```python
from build123d import *

# Parameters (mm, degrees)
BOSS_EXTRUDE1_DEPTH = 1.1
SKETCH3_W           = 2.15
SKETCH3_H           = 30
SKETCH4_W           = 2.15
SKETCH4_H           = 30
SKETCH5_R           = 1.5
CUT_EXTRUDE1_DEPTH  = 28


with BuildPart() as part:
    # Sketch2 → Boss-Extrude1 (new body)
    with BuildSketch(Plane.XY):
        with BuildLine():
            Line((-20.5, -0.55), (-13.5, -0.55))
            ThreePointArc((-13.5, -0.55), (-12.403984489, -0.096015511), (-11.95, 1))
            Line((-11.95, 1), (-11.95, 7))
            ThreePointArc((-11.95, 7), (-11, 7.95), (-10.05, 7))
            Line((-10.05, 7), (-10.05, 0))
            Line((-10.05, 0), (-10.05, -7))
            ThreePointArc((-10.05, -7), (-8, -9.05), (-5.95, -7))
            Line((-5.95, -7), (-5.95, 0))
            Line((-5.95, 0), (-5.95, 7))
            ThreePointArc((-5.95, 7), (-5, 7.95), (-4.05, 7))
            Line((-4.05, 7), (-4.05, 0))
            Line((-4.05, 0), (-4.05, -7))
            ThreePointArc((-4.05, -7), (-2, -9.05), (0.05, -7))
            Line((0.05, -7), (0.05, 0))
            Line((0.05, 0), (0.05, 7))
            ThreePointArc((0.05, 7), (1, 7.95), (1.95, 7))
            Line((1.95, 7), (1.95, 0))
            Line((1.95, 0), (1.95, -7))
            ThreePointArc((1.95, -7), (4, -9.05), (6.05, -7))
            Line((6.05, -7), (6.05, -1))
            ThreePointArc((6.05, -1), (6.181801948, -0.681801948), (6.5, -0.55))
            Line((6.5, -0.55), (13.5, -0.55))
            ThreePointArc((13.5, -0.55), (14.05, 0), (13.5, 0.55))
            Line((13.5, 0.55), (6.5, 0.55))
            ThreePointArc((6.5, 0.55), (5.403984489, 0.096015511), (4.95, -1))
            Line((4.95, -1), (4.95, -7))
            ThreePointArc((4.95, -7), (4, -7.95), (3.05, -7))
            Line((3.05, -7), (3.05, 0))
            Line((3.05, 0), (3.05, 7))
            ThreePointArc((3.05, 7), (1, 9.05), (-1.05, 7))
            Line((-1.05, 7), (-1.05, 0))
            Line((-1.05, 0), (-1.05, -7))
            ThreePointArc((-1.05, -7), (-2, -7.95), (-2.95, -7))
            Line((-2.95, -7), (-2.95, 0))
            Line((-2.95, 0), (-2.95, 7))
            ThreePointArc((-2.95, 7), (-5, 9.05), (-7.05, 7))
            Line((-7.05, 7), (-7.05, 0))
            Line((-7.05, 0), (-7.05, -7))
            ThreePointArc((-7.05, -7), (-8, -7.95), (-8.95, -7))
            Line((-8.95, -7), (-8.95, 0))
            Line((-8.95, 0), (-8.95, 7))
            ThreePointArc((-8.95, 7), (-11, 9.05), (-13.05, 7))
            Line((-13.05, 7), (-13.05, 1))
            ThreePointArc((-13.05, 1), (-13.181801948, 0.681801948), (-13.5, 0.55))
            Line((-13.5, 0.55), (-20.5, 0.55))
            ThreePointArc((-20.5, 0.55), (-21.05, 0), (-20.5, -0.55))
        make_face()
    extrude(amount=BOSS_EXTRUDE1_DEPTH)

    # Sketch3 → Revolve1 (revolve)
    with BuildSketch(Plane(origin=(0, 0, 0), x_dir=(-1, 0, 0), z_dir=(0, -1, 0)), mode=Mode.PRIVATE) as revolve1_sk:
        with Locations((21.575, 13.9)):
            Rectangle(SKETCH3_W, SKETCH3_H)
    revolve(revolve1_sk.sketch.rotate(Axis((-20.5, 0, 1.1), (0, 0, -1)), 180), axis=Axis((-20.5, 0, 1.1), (0, 0, -1)))

    # Sketch4 → Revolve2 (revolve)
    with BuildSketch(Plane(origin=(0, 0, 0), x_dir=(-1, 0, 0), z_dir=(0, -1, 0)), mode=Mode.PRIVATE) as revolve2_sk:
        with Locations((-14.575, 13.9)):
            Rectangle(SKETCH4_W, SKETCH4_H)
    revolve(revolve2_sk.sketch.rotate(Axis((13.5, 0, -28.9), (0, 0, 1)), 180), axis=Axis((13.5, 0, -28.9), (0, 0, 1)))

    # Sketch5 → Cut-Extrude1 (cut)
    with BuildSketch(Plane(origin=(0, 0, -28.9), x_dir=(-1, 0, 0), z_dir=(0, 0, -1))):
        with Locations((20.5, 0)):
            Circle(SKETCH5_R)
        with Locations((-13.5, 0)):
            Circle(SKETCH5_R)
    extrude(amount=-CUT_EXTRUDE1_DEPTH, mode=Mode.SUBTRACT)


solid = part.part
```
Can you work these out from the model? Positions are in its coordinate system, mm. A direction names the side the tool comes from. Give positions to 0.01 mm unless a question says otherwise; leave off trailing zeros. Order: outer loops, then holes, each group sorted by start corner. A loop starts at its lowest first (then second) coordinate and runs counter-clockwise, first axis right, second up. Notation, with made-up numbers: M -24.75,52.5 L -2.75,52.5 A21 ccw -2.75,86.5 Z; hole C 30.25,-11.5 d9. An arc over 180 degrees is marked long. One line per item, written item: value.
1) For P1, Ø2.5, axis at x = 13.5, y = 0, coming from the -Z side; P2, Ø0.9, axis at x = -16, z = 0.5, coming from the -Y side; P3, Ø0.6, axis at y = 0.5, z = 0.5, coming from the -X side; P4, Ø6, axis at x = 6.5, z = -7, coming from the +Y side, each with a flat end and sliding along its axis, tell me the tip position at first contact or that it passes through.
Answer sheet:
P1: stops at z = -0.9
P2: stops at y = -0.55
P3: stops at x = -22.64
P4: passes through
2) I want a section at A-A, the plane y = -2.75. List the corners of the cut face in (x, z) for me.
Answer sheet:
outline: M -10.05,0 L -8.95,0 L -8.95,1.1 L -10.05,1.1 Z; M -7.05,0 L -5.95,0 L -5.95,1.1 L -7.05,1.1 Z; M -4.05,0 L -2.95,0 L -2.95,1.1 L -4.05,1.1 Z; M -1.05,0 L 0.05,0 L 0.05,1.1 L -1.05,1.1 Z; M 1.95,0 L 3.05,0 L 3.05,1.1 L 1.95,1.1 Z; M 4.95,0 L 6.05,0 L 6.05,1.1 L 4.95,1.1 Z
3) I want a section at B-B, the plane z = -25.25. List the corners of the cut face in (x, y) for me.
Answer sheet:
outline: C -20.5,0 d4.3; C 13.5,0 d4.3; hole C -20.5,0 d3; hole C 13.5,0 d3
4) I want a section at D-D, the plane y = 7.5. List the corners of the cut face in (x, z) for me, plus the area to 3 significant figures.
Answer sheet:
outline: M -12.99,0 L -11.81,0 L -11.81,1.1 L -12.99,1.1 Z; M -10.19,0 L -9.01,0 L -9.01,1.1 L -10.19,1.1 Z; M -6.99,0 L -5.81,0 L -5.81,1.1 L -6.99,1.1 Z; M -4.19,0 L -3.01,0 L -3.01,1.1 L -4.19,1.1 Z; M -0.99,0 L 0.19,0 L 0.19,1.1 L -0.99,1.1 Z; M 1.81,0 L 2.99,0 L 2.99,1.1 L 1.81,1.1 Z
area: 7.79 mm^2
5) Please list where these lines run through material, in increasing order: line 1 along Y through (x, z) = (13.5, -11.5); line 2 along Z through (x, y) = (2.5, 0.25); line 3 along Y through (x, z) = (-21, -10.5).
Answer sheet:
line 1: y = -2.15 to -1.5, 1.5 to 2.15
line 2: z = 0 to 1.1
line 3: y = -2.09 to -1.41, 1.41 to 2.09
6) On a 3-axis mill with a long thin cutter (end or side, diameter ignored), from which of +Z, -Z, +X, -X, +Y, -Y can I reach the whole of each face in a straight line? I mean faces 3 (the face through (-2.95, -0.1, 0.5)), 4 (the face through (-19, 0, -15)), 5 (the face through (15, -1, -28.9)), 6 (the face through (6.05, -4, 0.5)). Say none if no direction works.
Answer sheet:
face 3: +Z, -Z, +Y
face 4: -Z
face 5: -Z, +X, -X, +Y, -Y
face 6: +Z, -Z, -Y
7) I want a section at C-C, the plane x = -5. List the corners of the cut face in (y, z) for me, plus the area to 3 significant figures.
Answer sheet:
outline: M 7.95,0 L 9.05,0 L 9.05,1.1 L 7.95,1.1 Z
area: 1.21 mm^2
8) We'd pull the mould along X, two halves only. Please class faces 1 (the face through (8.9, -0.55, 0.5)), 2 (the face through (-19, -1, -28.9)): released by +X, released by -X, zero draft, split by the parting line, or undercut.
Answer sheet:
face 1: undercut
face 2: zero draft
